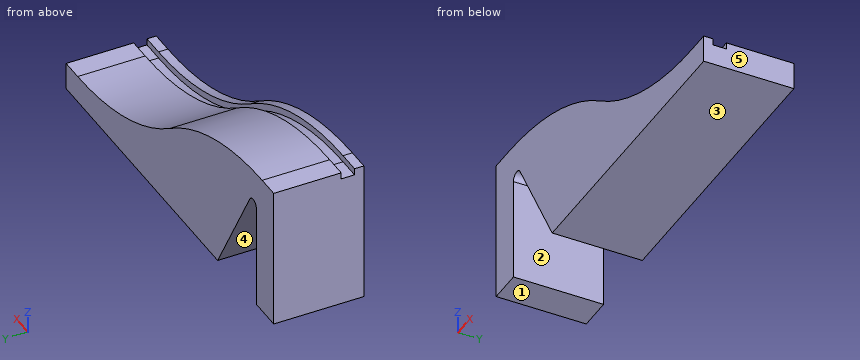
```python
from build123d import *

# Parameters (mm, degrees)
F1_DEPTH = 20.25
F2_W     = 6
F2_H     = 3


with BuildPart() as f1:
    # F0 (on Front) → F1 (new body, symmetric)
    with BuildSketch(Plane.XZ):
        with BuildLine():
            Line((10, 64.4), (0, 64.4))
            Line((0, 64.4), (0, 0))
            Line((0, 0), (15, 0))
            Line((15, 0), (15, 47))
            ThreePointArc((15, 47), (17.223543, 49.897777), (20.598076, 48.5))
            Line((20.598076, 48.5), (48.599564, 0))
            Line((48.599564, 0), (180, 0))
            Line((180, 0), (180, 12.4))
            Line((180, 12.4), (170, 12.4))
            ThreePointArc((170, 12.4), (127.940518, 19.063133), (90, 38.4))
            ThreePointArc((90, 38.4), (52.059482, 57.736867), (10, 64.4))
        make_face()
    extrude(amount=F1_DEPTH, both=True)

    # F3: sweep along a path in F0
    with BuildLine(Plane.XZ) as f3_path:
        Line((180, 12.4), (170, 12.4))
        ThreePointArc((170, 12.4), (127.940518, 19.063133), (90, 38.4))
        ThreePointArc((90, 38.4), (52.059482, 57.736867), (10, 64.4))
        Line((10, 64.4), (0, 64.4))
    # F2 (on face) → F3 (sweep, cut)
    with BuildSketch(Plane.YZ.offset(180)):
        with Locations((-13.075, 10.9)):
            Rectangle(F2_W, F2_H)
    sweep(path=f3_path.line, mode=Mode.SUBTRACT)


solid = f1.part
```
Geometry check sheet. Reference: the model listing, model coordinates, mm. Face numbers are marked on the shaded views. A direction names the side the tool comes from. Give positions to 0.01 mm unless a question says otherwise; leave off trailing zeros. Order: outer loops, then holes, each group sorted by start corner. A loop starts at its lowest first (then second) coordinate and runs counter-clockwise, first axis right, second up. Notation, with made-up numbers: (-28, 17.25) - (-14, 17.25) arc R13 cw to (-14, 29.25) - close; hole circle Ø9 at (63, 3.5). An arc over 180 degrees is marked (long way). Write item = value, one per line. Start each with the question number.
1) Section check D-D (z = 31). Enter the section's corners in (x, y) (3 decimals).
2) Scan lines: L1, parallel to X at y = -6, z = 8; L2, parallel to X at y = 19.5, z = 5.5; L3, parallel to Z at x = 11, y = 15.5. Record each from-to range of solid material in increasing order.
3) Section check B-B (z = 15.5). Enter the section's corners in (x, y) (3 decimals), then the cut area to 3 significant figures.
4) Draft check along X on the marked faces 3, 4 and 5. Enter one of: released by +X, released by -X, zero draft, split by the parting line, or undercut.
5) Section check C-C (x = 69). Enter the section's corners in (y, z) (3 decimals), then the cut area to 3 significant figures.
6) Access from +Z, -Z, +X, -X, +Y, -Y to the whole of each face (thin tool, end or side, straight path). Record for the marked faces 1 and 2.
7) Gauge pin test, flat ends, axial feed: pin 1 Ø5 at (x, y) = (174, 2) entering from +Z; pin 2 Ø1 at (y, z) = (-1, 30) entering from +X; pin 3 Ø1.8 at (x, y) = (177, -12) entering from +Z. Record the tip position at first contact, or that the pin passes through.
8) Section check A-A (y = 6.5). Enter the section's corners in (x, z).
Geometry check:
q1.outline = (0, -20.25) - (15, -20.25) - (15, 20.25) - (0, 20.25) - close; (30.702, -20.25) - (101.326, -20.25) - (101.326, -16.075) - (95.558, -16.075) - (95.558, -10.075) - (101.326, -10.075) - (101.326, 20.25) - (30.702, 20.25) - close
q2.L1 = 0 to 15, 43.98 to 180
q2.L2 = 0 to 15, 45.42 to 180
q2.L3 = 0 to 64.4
q3.outline = (0, -20.25) - (15, -20.25) - (15, 20.25) - (0, 20.25) - close; (39.651, -20.25) - (141.12, -20.25) - (141.12, -16.075) - (129.263, -16.075) - (129.263, -10.075) - (141.12, -10.075) - (141.12, 20.25) - (39.651, 20.25) - close
q3.area = 4,650 mm2
q4.face_3 = zero draft
q4.face_4 = undercut
q4.face_5 = released by +X
q5.outline = (-20.25, 0) - (20.25, 0) - (20.25, 50.944) - (-10.075, 50.944) - (-10.075, 47.606) - (-16.075, 47.606) - (-16.075, 50.944) - (-20.25, 50.944) - close
q5.area = 2,040 mm2
q6.face_1 = -Z, +X, -X, +Y, -Y
q6.face_2 = -Z, +Y, -Y
q7.pin_1 = 12.4
q7.pin_2 = 103.96
q7.pin_3 = 9.4
q8.outline = (0, 0) - (15, 0) - (15, 47) arc R3 cw to (20.6, 48.5) - (48.6, 0) - (180, 0) - (180, 12.4) - (170, 12.4) arc R136.08 cw to (90, 38.4) arc R136.08 ccw to (10, 64.4) - (0, 64.4) - close
